```python
from build123d import *

# Parameters (mm, degrees)
SKETCH_1_W               = 20
SKETCH_1_H               = 10
EXTRUDE_1_DEPTH          = 100
EXTRUDE_START            = -9
SKETCH_2_W               = 10
SKETCH_2_H               = 10
SKETCH_2_W_2             = 20
EXTRUDE_2_DEPTH          = 6
CUT_EXTRUDE_1_DEPTH      = 98.88258272
CUT_EXTRUDE_1_DEPTH_BACK = 98.88258272
SKETCH_3_R               = 2.5


with BuildPart() as part:
    # 草图1 → 凸台-拉伸1 (new body)
    with BuildSketch(Plane.XY):
        with Locations((10, 5)):
            Rectangle(SKETCH_1_W, SKETCH_1_H)
    extrude(amount=EXTRUDE_1_DEPTH)

    # 草图2 → 凸台-拉伸2 (add)
    with BuildSketch(Plane(origin=(0, 0, 0), x_dir=(-1, 0, 0), z_dir=(0, 0, -1)).offset(EXTRUDE_START)):
        with Locations((-25, 5)):
            Rectangle(SKETCH_2_W, SKETCH_2_H)
        with Locations((-10, 15)):
            Rectangle(SKETCH_2_W_2, SKETCH_2_H)
        with Locations((5, 5)):
            Rectangle(SKETCH_2_W, SKETCH_2_H)
    extrude_2 = extrude(amount=-EXTRUDE_2_DEPTH)

    # 镜向1: 凸台-拉伸2 across plane
    add(extrude_2.mirror(Plane(origin=(0, 0, 50), x_dir=(1, 0, 0), z_dir=(0, 0, -1))))

    # 草图3 → 切除-拉伸1 (cut, two sides: drawn at the far end of the back side and taken through both)
    with BuildSketch(Plane(origin=(0, 0, 9), x_dir=(-1, 0, 0), z_dir=(0, 0, -1)).offset(-CUT_EXTRUDE_1_DEPTH_BACK)):
        with Locations(Location((5, 5, 0), (0, 0, 180))):
            Circle(SKETCH_3_R)
        with Locations(Location((-10, 15, 0), (0, 0, 180))):
            Circle(SKETCH_3_R)
        with Locations(Location((-25, 5, 0), (0, 0, 180))):
            Circle(SKETCH_3_R)
    extrude(amount=CUT_EXTRUDE_1_DEPTH + CUT_EXTRUDE_1_DEPTH_BACK, mode=Mode.SUBTRACT)


solid = part.part
```
Geometry check sheet. Reference: the model listing, model coordinates, mm. A direction names the side the tool comes from. Coordinates: 2 decimals unless noted, no trailing zeros. Order: outer loops, then holes, each group sorted by start corner. A loop starts at its lowest first (then second) coordinate and runs counter-clockwise, first axis right, second up. Notation, with made-up numbers: M 70,70 L 91,70 A9 ccw 91,81 Z; hole C 51.5,4 d7. An arc over 180 degrees is marked long. Answer as a JSON object with one key per item and string values.
Q1. Cross-section at C-C on y = 15. Record the cut outline in (x, z).
Results are:
{"outline": "M 0,9 L 7.5,9 L 7.5,15 L 0,15 Z; M 0,85 L 7.5,85 L 7.5,91 L 0,91 Z; M 12.5,9 L 20,9 L 20,15 L 12.5,15 Z; M 12.5,85 L 20,85 L 20,91 L 12.5,91 Z"}
Q2. Cross-section at B-B on x = -3.5. Record the cut outline in (y, z), and give its area (3 significant figures).
Results are:
{"outline": "M 0,9 L 3,9 L 3,15 L 0,15 Z; M 0,85 L 3,85 L 3,91 L 0,91 Z; M 7,9 L 10,9 L 10,15 L 7,15 Z; M 7,85 L 10,85 L 10,91 L 7,91 Z", "area": "72.0 mm²"}
Q3. Scan lines: line 1 (Z direction, x = 12, y = 17.5); line 2 (Y direction, x = 25, z = 13.85); line 3 (Y direction, x = 10, z = 12). Record each from-to range of solid material in increasing order.
Results are:
{"line 1": "z = 9 to 15, 85 to 91", "line 2": "y = 0 to 2.5, 7.5 to 10", "line 3": "y = 0 to 12.5, 17.5 to 20"}
Q4. Cross-section at A-A on x = 8.5. Record the cut outline in (y, z), and give its area (3 significant figures).
Results are:
{"outline": "M 0,0 L 10,0 L 10,9 L 13,9 L 13,15 L 10,15 L 10,85 L 13,85 L 13,91 L 10,91 L 10,100 L 0,100 Z; M 17,9 L 20,9 L 20,15 L 17,15 Z; M 17,85 L 20,85 L 20,91 L 17,91 Z", "area": "1,070 mm²"}
Q5. Depth check by flat-ended pin: pin 1 Ø11 at (x, y) = (27, 3) entering from +Z; pin 2 Ø5 at (y, z) = (16.5, 12) entering from -X; pin 3 Ø6 at (x, z) = (14, 62.5) entering from +Y; pin 4 Ø4.5 at (x, y) = (10, 15) entering from -Z. Enter the tip coordinate at first touch or a pass-through.
Results are:
{"pin 1": "stops at z = 91", "pin 2": "stops at x = 0", "pin 3": "stops at y = 10", "pin 4": "passes through"}
Q6. Release check for a two-part mould opening along Z. For faces 4 (the flat face through (20, 15, 12)), 5 (the flat face through (12.4, 16.2, 15)), 6 (the flat face through (-3, 7, 91)), 7 (the flat face through (12.4, 16.2, 85)) record: released by +Z, released by -Z, zero draft, split by the parting line, or undercut.
Results are:
{"face 4": "zero draft", "face 5": "undercut", "face 6": "released by +Z", "face 7": "undercut"}
Q7. Cross-section at D-D on y = 9. Record the cut outline in (x, z).
Results are:
{"outline": "M -10,9 L 0,9 L 0,0 L 20,0 L 20,9 L 30,9 L 30,15 L 20,15 L 20,85 L 30,85 L 30,91 L 20,91 L 20,100 L 0,100 L 0,91 L -10,91 L -10,85 L 0,85 L 0,15 L -10,15 Z"}
Q8. Tool access check on faces 1 (the flat face through (10, 10, 4)), 2 (the flat face through (20, 5, 50)), 3 (the flat face through (-3, 7, 85)). Record the directions out of +Z, -Z, +X, -X, +Y, -Y that give a thin tool (end or side, any length) a straight path to the whole face; none if there is none.
Results are:
{"face 1": "-Z, +X, -X, +Y", "face 2": "+X, +Y, -Y", "face 3": "-X, +Y, -Y"}
